from build123d import *

# Parameters (mm, degrees)
BOSS_EXTRUDE1_DEPTH = 200
CIRPATTERN1_COUNT   = 4
FILLET1_R           = 50


with BuildPart() as part:
    # Sketch1 → Boss-Extrude1 (new body)
    with BuildSketch(Plane(origin=(0, 0, 0), x_dir=(0, 1, 0), z_dir=(0, 0, 1))):
        with BuildLine():
            Line((-50, 141.421356237), (-50, 0))
            Line((-50, 0), (50, 0))
            Line((50, 0), (50, 141.421356237))
            ThreePointArc((50, 141.421356237), (0, 150), (-50, 141.421356237))
        make_face()
    extrude(amount=BOSS_EXTRUDE1_DEPTH)


with BuildPart() as cirpattern1_1:
    # CirPattern1: pattern copy
    add(part.part.rotate(Axis((0, 0, 0), (0, 0, 1)), 1 * 360 / CIRPATTERN1_COUNT))


with BuildPart() as cirpattern1_2:
    # CirPattern1: pattern copy
    add(part.part.rotate(Axis((0, 0, 0), (0, 0, 1)), 2 * 360 / CIRPATTERN1_COUNT))


with BuildPart() as cirpattern1_3:
    # CirPattern1: pattern copy
    add(part.part.rotate(Axis((0, 0, 0), (0, 0, 1)), 3 * 360 / CIRPATTERN1_COUNT))


with BuildPart() as part_1:
    add(part.part)

    # Combine1: union CirPattern1_1, CirPattern1_2, CirPattern1_3
    add(cirpattern1_1.part)
    add(cirpattern1_2.part)
    add(cirpattern1_3.part)

    # Fillet1
    fillet1_edges = [part_1.edges().sort_by_distance(p)[0] for p in [
        (-50, 50, 100),
        (-50, -50, 100),
        (50, -50, 100),
        (50, 50, 100),
    ]]
    fillet(fillet1_edges, radius=FILLET1_R)


solid = part_1.part
The listing builds one solid part. Answer for the finished solid, in the listing's coordinates (mm). A direction names the side the tool comes from. Coordinates: 2 decimals unless noted, no trailing zeros. Write each loop counter-clockwise with the first axis right and the second up, starting at its lowest first coordinate (ties: lowest second). Pieces come first, ordered by that corner, then holes. Notation, with made-up numbers: (47, -29.75) - (93, -29.75) arc R9 ccw to (93, -21.75) - close; hole circle Ø10 at (-32, 69.25). An arc over 180 degrees is marked (long way). Answer as CSV lines item,"result".
1. Find section A-A (z = 116.5). Give the vertices of the cut face in (x, y).
Computed values:
outline,"(-141.42, -50) - (-100, -50) arc R50 cw to (-50, -100) - (-50, -141.42) arc R150 ccw to (50, -141.42) - (50, -100) arc R50 cw to (100, -50) - (141.42, -50) arc R150 ccw to (141.42, 50) - (100, 50) arc R50 cw to (50, 100) - (50, 141.42) arc R150 ccw to (-50, 141.42) - (-50, 100) arc R50 cw to (-100, 50) - (-141.42, 50) arc R150 ccw to start"
2. Find section B-B (y = 110.5). Give the vertices of the cut face in (x, z), plus the area to 3 significant figures.
Computed values:
outline,"(-50, 0) - (50, 0) - (50, 200) - (-50, 200) - close"
area,"20,000 mm²"
3. A tool of negligible diameter and unlimited length cuts with its end or side. For faces 1 (the flat face through (-50, 121, 99)), 2 (the flat face through (-50, -120, 99)), 3 (the flat face through (120, -50, 99)), 4 (the flat face through (50, 120, 99)), from which of +Z, -Z, +X, -X, +Y, -Y can it reach the whole face along a straight path? Write none if from no direction.
Computed values:
face 1,"+Z, -Z, -X, +Y"
face 2,"+Z, -Z, -X, -Y"
face 3,"+Z, -Z, +X, -Y"
face 4,"+Z, -Z, +X, +Y"
4. Given P1, Ø12.5, axis at x = 111.5, z = 88, coming from the -Y side; P2, Ø12, axis at y = -75.5, z = 54, coming from the -X side; P3, Ø2, axis at x = -58.5, z = 86.5, coming from the -Y side, each flat-ended and moving along its own axis, determine where each tip first touches the part or whether it passes through.
Computed values:
P1,"stops at y = -50"
P2,"stops at x = -60.38"
P3,"stops at y = -73.66"
5. Straight lines are drawn through the part: line 1 (X direction, y = -136, z = 70.5); line 2 (Y direction, x = 89.5, z = 188). For each, find the intervals that lie inside material, in ascending order. Write a range as [from, to].
Computed values:
line 1,"x = [-50, 50]"
line 2,"y = [-51.11, 51.11]"
